Autodesk Fusion 360 part; units mm, degrees
sketch "Sketch1" plane through (0, 0, 0) normal (0, 1, 0) x (1, 0, 0)
  line L0 (12.4312, -14.3607) -> (13.4312, -14.3607)
  line L1 (13.4312, -14.3607) -> (13.4312, -17.3607)
  line L2 (13.4312, -17.3607) -> (12.4312, -17.3607)
  line L3 (12.4312, -17.3607) -> (12.4312, -14.3607)
  line L4 (12.9312, -14.3607) -> (12.9312, -17.3607) construction
  line L5 (12.4312, -15.8607) -> (13.4312, -15.8607) construction
  line L6 (13.4312, -15.8607) -> (18.2312, -15.8607) construction
  line L7 (18.2312, -14.3607) -> (18.2312, -17.3607) construction
  line L8 (17.7312, -14.3607) -> (18.7312, -14.3607)
  line L9 (18.7312, -14.3607) -> (18.7312, -17.3607)
  line L10 (18.7312, -17.3607) -> (17.7312, -17.3607)
  line L11 (17.7312, -17.3607) -> (17.7312, -14.3607)
  line L12 (9.8312, -10.8607) -> (21.8312, -10.8607)
  line L13 (21.8312, -10.8607) -> (21.8312, -22.2607)
  line L14 (21.8312, -22.2607) -> (9.8312, -22.2607)
  line L15 (9.8312, -22.2607) -> (9.8312, -10.8607)
  line L16 (15.8312, -10.8607) -> (15.8312, -22.2607) construction
  line L17 (21.8312, -16.5607) -> (9.8312, -16.5607) construction
  line L18 (10.0312, -12.2607) -> (21.6312, -12.2607)
  line L19 (21.6312, -12.2607) -> (21.6312, -20.8607)
  line L20 (21.6312, -20.8607) -> (10.0312, -20.8607)
  line L21 (10.0312, -20.8607) -> (10.0312, -12.2607)
  line L22 (10.8012, -13.0307) -> (20.8612, -13.0307)
  line L23 (20.8612, -13.0307) -> (20.8612, -20.0907)
  line L24 (20.8612, -20.0907) -> (10.8012, -20.0907)
  line L25 (10.8012, -20.0907) -> (10.8012, -13.0307)
  point P0 (15.8312, -15.8607)
  point P1 (21.6312, -16.5607)
  point P2 (15.8312, -12.2607)
  dimension "d3" = 1
  dimension "d4" = 3
  dimension "d6" = 1
  dimension "d7" = 3
  dimension "d8" = 5.3
  dimension "d9" = 12
  dimension "d10" = 11.4
  dimension "d11" = 5
  dimension "d14" = 11.6
  dimension "d15" = 8.6
  dimension "d17" = 0.77
  dimension "d18" = 0.77
  dimension "d19" = 0.77
  dimension "d20" = 0.77
extrude "Extrude1" add sketch "Sketch1" along normal blind 2 contours L0 L1 L2 L3 | L8 L9 L10 L11 makes body 1 at (13.4312, 0.6667, 15.3607) makes body 2 at (18.7312, 0.6667, 15.3607)
extrude "Extrude2" add sketch "Sketch1" along normal blind 5 from surface at 2 contours L0 L1 L2 L3 | L8 L9 L10 L11 | L22 L23 L24 L25 bodies 1 2
fillet "Fillet1" [suppressed]
sketch "Sketch2" plane through (0, 7, 0) normal (0, 1, 0) x (-1, 0, 0)
  line L0 (-16.9627, 13.8658) -> (-16.9627, 19.7076) construction
  line L1 (-16.9627, 19.7076) -> (-20.9627, 19.7076) construction
  line L2 (-20.9627, 19.7076) -> (-20.9627, 13.8658) construction
  line L3 (-20.9627, 13.8658) -> (-16.9627, 13.8658) construction
  line L4 (-11.5741, 13.8658) -> (-11.5741, 19.7076) construction
  line L5 (-11.5741, 19.7076) -> (-15.5741, 19.7076) construction
  line L6 (-15.5741, 19.7076) -> (-15.5741, 13.8658) construction
  line L7 (-15.5741, 13.8658) -> (-11.5741, 13.8658) construction
  line L8 (-10.8012, 13.0307) -> (-10.8012, 20.0907)
  line L9 (-10.8012, 20.0907) -> (-20.8612, 20.0907)
  line L10 (-20.8612, 20.0907) -> (-20.8612, 13.0307)
  line L11 (-20.8612, 13.0307) -> (-10.8012, 13.0307)
extrude "Extrude3" [suppressed]
extrude "Extrude4" [suppressed]
equation "PostW = 1 mm"
equation "PostH = 3 mm"
equation "d3 = PostW"
equation "d4 = PostH"
equation "d6 = PostW"
equation "d7 = PostH"
equation "HoleW = 8.6 mm"
equation "HoleH = 11.6 mm"
equation "d14 = HoleH"
equation "d15 = HoleW"
equation "HoleTol = 0.77 mm"
equation "d17 = HoleTol"
equation "d18 = HoleTol"
equation "d19 = HoleTol"
equation "d20 = HoleTol"
equation "CapD = 5 mm"
equation "PostD = 2 mm"
equation "d23 = PostD"
equation "d26 = CapD"
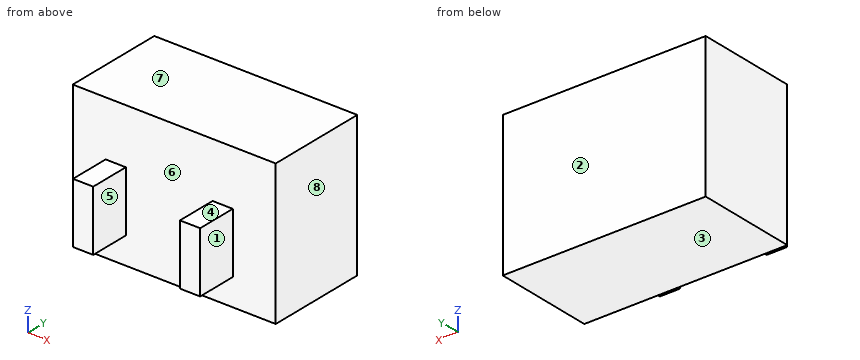
Check sheet for the modelled part. Datum: model origin and axes. Units: mm. Face numbers are marked on the shaded views. A direction names the side the tool comes from. Round coordinates to 2 decimals unless told otherwise and drop trailing zeros. Loops run counter-clockwise (first coordinate to the right, second up) from the corner with the lowest first, then second, coordinate; pieces in that order, holes last. Notation, with made-up numbers: M 72,43 L 83,43 A27 ccw 83,62 Z; hole C 36.5,-11 d7. An arc over 180 degrees is marked long. Answer as a JSON object with one key per item and string values.
1. Mould release check, pull along X, two halves, no side actions. Record for the marked faces 6, 7 and 8: pulls with the +X half, pulls with the -X half, needs draft (parallel to the pull), parting line crosses it, or undercut.
Reply:
{"face 6": "undercut", "face 7": "needs draft", "face 8": "pulls with the +X half"}
2. Scan lines: line 1 (X direction, y = 1.75, z = 16.5); line 2 (Y direction, x = 17, z = 16); line 3 (Z direction, x = 12.75, y = 0.5). Record each from-to range of solid material in increasing order.
Reply:
{"line 1": "x = 12.43 to 13.43, 17.73 to 18.73", "line 2": "y = 2 to 7", "line 3": "z = 14.36 to 17.36"}
3. Gauge pin test, flat ends, axial feed: P1, Ø1.6, axis at y = 0.5, z = 15.5, coming from the -X side; P2, Ø1.1, axis at x = 13, y = 1, coming from the -Z side; P3, Ø1.1, axis at x = 18.5, y = 0.5, coming from the +Z side. Record the tip position at first contact, or that the pin passes through.
Reply:
{"P1": "stops at x = 12.43", "P2": "stops at z = 14.36", "P3": "stops at z = 17.36"}
4. Access from +Z, -Z, +X, -X, +Y, -Y to the whole of each face (thin tool, end or side, straight path). Record for the marked faces 1, 2, 3, 4 and 5.
Reply:
{"face 1": "+Z, -Z, +X, -Y", "face 2": "+Z, -Z, +X, -X, +Y", "face 3": "-Z, +X, -X, +Y, -Y", "face 4": "+Z, +X, -X, -Y", "face 5": "+Z, -Z, -Y"}
5. Section check B-B (z = 14.5). Record the boundary of the cut face in (x, y).
Reply:
{"outline": "M 10.8,2 L 12.43,2 L 12.43,0 L 13.43,0 L 13.43,2 L 17.73,2 L 17.73,0 L 18.73,0 L 18.73,2 L 20.86,2 L 20.86,7 L 10.8,7 Z"}
6. Section check A-A (y = 1.5). Record the boundary of the cut face in (x, z).
Reply:
{"outline": "M 12.43,14.36 L 13.43,14.36 L 13.43,17.36 L 12.43,17.36 Z; M 17.73,14.36 L 18.73,14.36 L 18.73,17.36 L 17.73,17.36 Z"}
7. Section check C-C (x = 18.5). Record the boundary of the cut face in (y, z).
Reply:
{"outline": "M 0,14.36 L 2,14.36 L 2,13.03 L 7,13.03 L 7,20.09 L 2,20.09 L 2,17.36 L 0,17.36 Z"}
8. Section check D-D (z = 17.5). Record the boundary of the cut face in (x, y), plus the area to 3 significant figures.
Reply:
{"outline": "M 10.8,2 L 20.86,2 L 20.86,7 L 10.8,7 Z", "area": "50.3 mm²"}
